Input: part model. Units: mm. Frame: model coordinates. Face numbers are marked on the shaded views. A direction names the side the tool comes from. Coordinates: 2 decimals unless noted, no trailing zeros. Loops run counter-clockwise (first coordinate to the right, second up) from the corner with the lowest first, then second, coordinate; pieces in that order, holes last.
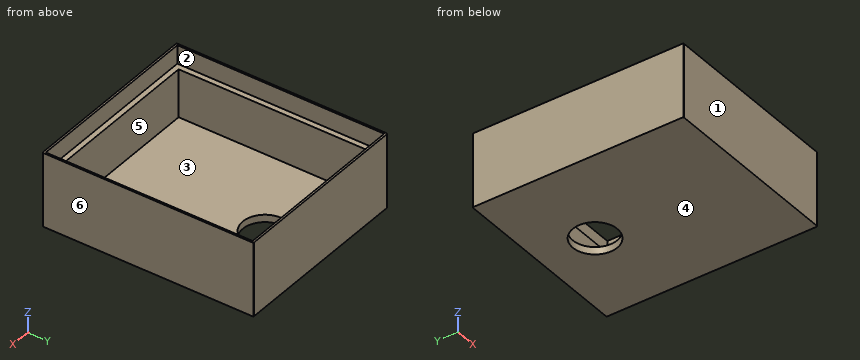
```python
from build123d import *

# Parameters (mm, degrees)
EXTRUDE_1_DEPTH     = 200
SHELL_1_T           = -20
CUT_EXTRUDE_1_DEPTH = 50
SKETCH_3_R          = 60
CUT_EXTRUDE_2_DEPTH = 50


with BuildPart() as part:
    # 草图1 → 凸台-拉伸1 (new body)
    with BuildSketch(Plane.XY):
        with BuildLine():
            Line((3, 0), (497, 0))
            ThreePointArc((497, 0), (499.121320344, -0.878679656), (500, -3))
            Line((500, -3), (500, -567))
            ThreePointArc((500, -567), (499.121320344, -569.121320344), (497, -570))
            Line((497, -570), (3, -570))
            ThreePointArc((3, -570), (0.878679656, -569.121320344), (0, -567))
            Line((0, -567), (0, -3))
            ThreePointArc((0, -3), (0.878679656, -0.878679656), (3, 0))
        make_face()
    extrude(amount=EXTRUDE_1_DEPTH)

    # 抽壳1
    shell_1_openings = [part.faces().sort_by_distance(p)[0] for p in [
        (250, -285, 200),
    ]]
    offset(amount=SHELL_1_T, openings=shell_1_openings, kind=Kind.INTERSECTION)

    # 草图2 → 切除-拉伸1 (cut)
    with BuildSketch(Plane.XY.offset(200)):
        Polygon((4.785, -5.49), (495.215, -5.49), (495.215, -20), (495.215, -550), (495.215, -564.51), (4.785, -564.51), (4.785, -550), (4.785, -20), align=None)
    extrude(amount=-CUT_EXTRUDE_1_DEPTH, mode=Mode.SUBTRACT)

    # 草图3 → 切除-拉伸2 (cut)
    with BuildSketch(Plane(origin=(0, 0, 0), x_dir=(-1, 0, 0), z_dir=(0, 0, -1))):
        with Locations((-250, -150)):
            Circle(SKETCH_3_R)
    extrude(amount=-CUT_EXTRUDE_2_DEPTH, mode=Mode.SUBTRACT)


solid = part.part
```
Item 1: Reachability of the marked faces 1 and 2 from +Z, -Z, +X, -X, +Y, -Y: full face, straight path, thin tool, end or side. Return the list, or none.
Result:
face 1: +Z, -Z, +X, -X, -Y
face 2: +Z
Item 2: Section query A-A (y = -150). Output: boundary loops of the cut face in (x, z) (3 decimals), then the cut area to 3 significant figures.
Result:
outline: (0, 0) - (190, 0) - (190, 20) - (20, 20) - (20, 150) - (4.785, 150) - (4.785, 200) - (0, 200) - close; (310, 0) - (500, 0) - (500, 200) - (495.215, 200) - (495.215, 150) - (480, 150) - (480, 20) - (310, 20) - close
area: 13,300 mm2
Item 3: Section query C-C (z = 136). Output: boundary loops of the cut face in (x, y), then the cut area to 3 significant figures.
Result:
outline: (0, -567) arc R3 ccw to (3, -570) - (497, -570) arc R3 ccw to (500, -567) - (500, -3) arc R3 ccw to (497, 0) - (3, 0) arc R3 ccw to (0, -3) - close; hole (20, -550) - (480, -550) - (480, -20) - (20, -20) - close
area: 41,200 mm2
Item 4: Section query D-D (x = 102). Output: boundary loops of the cut face in (y, z).
Result:
outline: (-570, 0) - (0, 0) - (0, 200) - (-5.49, 200) - (-5.49, 150) - (-20, 150) - (-20, 20) - (-550, 20) - (-550, 150) - (-564.51, 150) - (-564.51, 200) - (-570, 200) - close
Item 5: Line query: L1, parallel to X at y = -204, z = 169.5 (3 decimals); L2, parallel to Y at x = 244, z = 187; L3, parallel to Y at x = 230, z = 121.5. Output: solid intervals per line, ascending.
Result:
L1: x = 0 to 4.785, 495.215 to 500
L2: y = -570 to -564.51, -5.49 to 0
L3: y = -570 to -550, -20 to 0
Item 6: Mould query, pull axis X, two halves, no side actions, for the marked faces 3, 4, 5 and 6. Classes: +X half, -X half, draft (parallel to the pull), parting line (faces both ways), or undercut.
Result:
face 3: undercut
face 4: draft
face 5: undercut
face 6: +X half
Item 7: Contact query for flat-ended pins moving along their axis: P1, Ø12, axis at x = 56, y = -268.5, coming from the +Z side; P2, Ø2, axis at x = 273.5, y = -258, coming from the -Z side. Output: stop coordinate, or through.
Result:
P1: stops at z = 20
P2: stops at z = 0
Item 8: Section query B-B (x = 250). Output: boundary loops of the cut face in (y, z), then the cut area to 3 significant figures.
Result:
outline: (-570, 0) - (-210, 0) - (-210, 20) - (-550, 20) - (-550, 150) - (-564.51, 150) - (-564.51, 200) - (-570, 200) - close; (-90, 0) - (0, 0) - (0, 200) - (-5.49, 200) - (-5.49, 150) - (-20, 150) - (-20, 20) - (-90, 20) - close
area: 14,700 mm2
